Input: part model. Units: mm. Frame: model coordinates. Face numbers are marked on the shaded views. A direction names the side the tool comes from. Round coordinates to 2 decimals unless told otherwise and drop trailing zeros. Loops run counter-clockwise (first coordinate to the right, second up) from the corner with the lowest first, then second, coordinate; pieces in that order, holes last. Notation, with made-up numbers: (-8.5, 82.25) - (22.5, 82.25) arc R36 cw to (22.5, 118.25) - close; hole circle Ø6 at (-32.5, 74). An arc over 180 degrees is marked (long way). Use CSV: the item, a comma, the result in double quotes. Start each with the question number.
1. Pull-direction query (Z, two-part tool) for the marked faces 1, 2, 3 and 4; classes: +Z half, -Z half, draft (parallel to the pull), parting line (faces both ways), or undercut.
2. Material intervals for probe 1 along Z at (x, y) = (-7, 2.75); probe 2 along X at (y, z) = (-5.75, 2.25); probe 3 along Z at (x, y) = (23, -7.5), sorted ascending. Write a range as from..to.
3. Cut plane B-B (z = -1). Return loops of the section in (x, y), and give its area (3 significant figures).
4. Cut plane A-A (y = 6.5). Return loops of the section in (x, z), and give its area (3 significant figures).
5. Access query for the marked faces 5, 6, 7 and 8. Directions: +Z, -Z, +X, -X, +Y, -Y. A direction counts if a zero-diameter tool reaches every point of the face in a straight line with its end or side. Return the directions, or none.
6. Pin query (flat end, axial travel): P1, Ø10, axis at x = 20, y = 8.5, coming from the -Z side; P2, Ø11, axis at x = -4, y = 2, coming from the -Z side; P3, Ø0.6, axis at x = -8, z = 3.5, coming from the +Y side. Return the tip coordinate at first contact, or that it passes through.
7. Cut plane D-D (z = 9). Return loops of the section in (x, y), and give its area (3 significant figures).
8. Cut plane C-C (y = 0). Return loops of the section in (x, z), and give its area (3 significant figures).
```python
from build123d import *

# Parameters (mm, degrees)
F0_R     = 11
F0_R_2   = 1.5
F1_DEPTH = 25
F2_R     = 12.5
F2_R_2   = 10
F3_DEPTH = 3
F4_W     = 10
F4_H     = 2
F4_H_2   = 2.5
F5_DEPTH = 12


with BuildPart() as f1:
    # F0 (on Right) → F1 (new body)
    with BuildSketch(Plane.YZ):
        Circle(F0_R)
        with Locations((-6.5, 0)):
            Circle(F0_R_2, mode=Mode.SUBTRACT)
        with Locations((6.5, 0)):
            Circle(F0_R_2, mode=Mode.SUBTRACT)
    extrude(amount=F1_DEPTH)

    # F2 (on face) → F3 (cut)
    with BuildSketch(Plane(origin=(0, 0, 0), x_dir=(0, -1, 0), z_dir=(-1, 0, 0))):
        Circle(F2_R)
        Circle(F2_R_2, mode=Mode.SUBTRACT)
    extrude(amount=-F3_DEPTH, mode=Mode.SUBTRACT)

    # F4 (on face) → F5 (join)
    with BuildSketch(Plane(origin=(0, 0, 0), x_dir=(0, -1, 0), z_dir=(-1, 0, 0))):
        with Locations((0, 4)):
            Rectangle(F4_W, F4_H)
        with Locations((0, -7.25)):
            Rectangle(F4_W, F4_H_2)
    extrude(amount=F5_DEPTH)


solid = f1.part
```
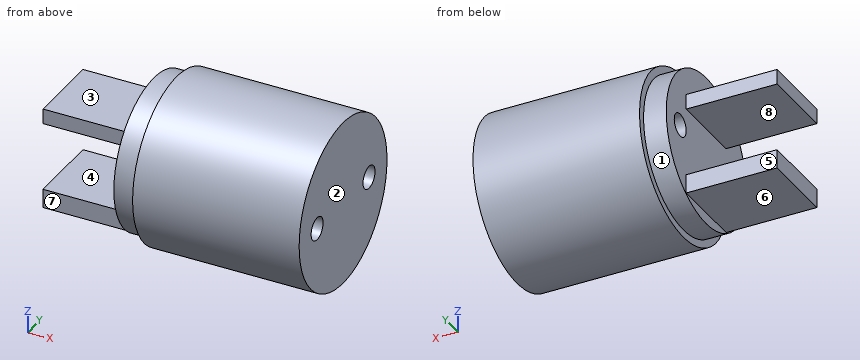
Established:
1,face 1,"parting line"
1,face 2,"draft"
1,face 3,"+Z half"
1,face 4,"undercut"
2,probe 1,"z = -8.5..-6, 3..5"
2,probe 2,"x = 0..25"
2,probe 3,"z = -8.05..-1.12, 1.12..8.05"
3,outline,"(0, -9.95) - (3, -9.95) - (3, -10.95) - (25, -10.95) - (25, -7.62) - (0, -7.62) - close; (0, -5.38) - (25, -5.38) - (25, 5.38) - (0, 5.38) - close; (0, 7.62) - (25, 7.62) - (25, 10.95) - (3, 10.95) - (3, 9.95) - (0, 9.95) - close"
3,area,"430 mm2"
4,outline,"(0, -7.6) - (3, -7.6) - (3, -8.87) - (25, -8.87) - (25, -1.5) - (0, -1.5) - close; (0, 1.5) - (25, 1.5) - (25, 8.87) - (3, 8.87) - (3, 7.6) - (0, 7.6) - close"
4,area,"361 mm2"
5,face 5,"+Z, -Z, -X, +Y"
5,face 6,"-Z, -X, +Y, -Y"
5,face 7,"+Z, -Z, -X, -Y"
5,face 8,"-X, +Y, -Y"
6,P1,"stops at z = -10.43"
6,P2,"stops at z = -10"
6,P3,"stops at y = 5"
7,outline,"(0, -4.36) - (3, -4.36) - (3, -6.32) - (25, -6.32) - (25, 6.32) - (3, 6.32) - (3, 4.36) - (0, 4.36) - close"
7,area,"304 mm2"
8,outline,"(-12, -8.5) - (0, -8.5) - (0, -10) - (3, -10) - (3, -11) - (25, -11) - (25, 11) - (3, 11) - (3, 10) - (0, 10) - (0, 5) - (-12, 5) - (-12, 3) - (0, 3) - (0, -6) - (-12, -6) - close"
8,area,"598 mm2"
